```python
from build123d import *

# Parameters (mm, degrees)
F0_W     = 106.52008
F0_H     = 110.235908
F1_DEPTH = 96.774
F2_R     = 26.380543
F3_DEPTH = 130.81
F4_R     = 5.08


with BuildPart() as f1:
    # F0 (on Top) → F1 (new body)
    with BuildSketch(Plane.XY):
        Rectangle(F0_W, F0_H)
    extrude(amount=F1_DEPTH)

    # F2 (on face) → F3 (cut)
    with BuildSketch(Plane.XY.offset(96.774)):
        Circle(F2_R)
    extrude(amount=-F3_DEPTH, mode=Mode.SUBTRACT)

    # F4
    f4_edges = [f1.edges().sort_by_distance(p)[0] for p in [
        (0, 55.117954, 96.774),
        (-53.26004, 0, 96.774),
        (0, -55.117954, 96.774),
        (53.26004, 0, 96.774),
        (53.26004, -55.117954, 48.387),
        (-53.26004, -55.117954, 48.387),
        (0, -55.117954, 0),
        (-53.26004, 0, 0),
        (-53.26004, 55.117954, 48.387),
        (0, 55.117954, 0),
        (53.26004, 55.117954, 48.387),
        (53.26004, 0, 0),
    ]]
    fillet(f4_edges, radius=F4_R)


solid = f1.part
```
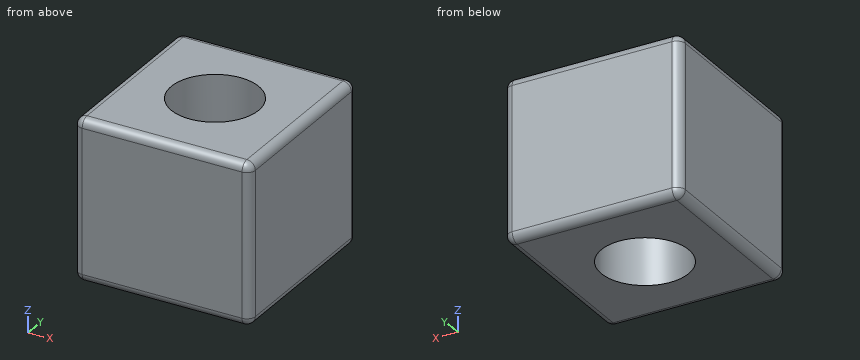
Verification items for the finished model (mm, model axes). Coordinates: 2 decimals unless noted, no trailing zeros. Write each loop counter-clockwise with the first axis right and the second up, starting at its lowest first coordinate (ties: lowest second). Pieces come first, ordered by that corner, then holes. Notation, with made-up numbers: (62, 23) - (92, 23) arc R15 ccw to (92, 39) - close; hole circle Ø4 at (65, 19.5). An arc over 180 degrees is marked (long way). One line per question, with ' | ' between items. Start each with the question number.
1. Section check A-A (z = 88). Enter the section's corners in (x, y), plus the area to 3 significant figures.
2. Section check B-B (x = 0). Enter the section's corners in (y, z), plus the area to 3 significant figures.
3. Material ranges on line 1 along Y through (x, z) = (0, 21); line 2 along X through (y, z) = (50.5, 55.5); line 3 along X through (y, z) = (-8, 53.5), recorded low to high.
4. Section check C-C (y = 0). Enter the section's corners in (x, z).
Computed values:
1) outline: (-53.26, -50.04) arc R5.08 ccw to (-48.18, -55.12) - (48.18, -55.12) arc R5.08 ccw to (53.26, -50.04) - (53.26, 50.04) arc R5.08 ccw to (48.18, 55.12) - (-48.18, 55.12) arc R5.08 ccw to (-53.26, 50.04) - close; hole circle Ø52.76 at (0, 0) | area: 9,530 mm²
2) outline: (-55.12, 5.08) arc R5.08 ccw to (-50.04, 0) - (-26.38, 0) - (-26.38, 96.77) - (-50.04, 96.77) arc R5.08 ccw to (-55.12, 91.69) - close; (26.38, 0) - (50.04, 0) arc R5.08 ccw to (55.12, 5.08) - (55.12, 91.69) arc R5.08 ccw to (50.04, 96.77) - (26.38, 96.77) - close | area: 5,540 mm²
3) line 1: -55.12 to -26.38, 26.38 to 55.12 | line 2: -53.24 to 53.24 | line 3: -53.26 to -25.14, 25.14 to 53.26
4) outline: (-53.26, 5.08) arc R5.08 ccw to (-48.18, 0) - (-26.38, 0) - (-26.38, 96.77) - (-48.18, 96.77) arc R5.08 ccw to (-53.26, 91.69) - close; (26.38, 0) - (48.18, 0) arc R5.08 ccw to (53.26, 5.08) - (53.26, 91.69) arc R5.08 ccw to (48.18, 96.77) - (26.38, 96.77) - close
